CAD build for the part. Positions are in the model's coordinates, mm. Face numbers are marked on the shaded views. A direction names the side the tool comes from. Round coordinates to 2 decimals unless told otherwise and drop trailing zeros. Loops run counter-clockwise (first coordinate to the right, second up) from the corner with the lowest first, then second, coordinate; pieces in that order, holes last. Notation, with made-up numbers: M 87.5,22.25 L 135.5,22.25 A17 cw 135.5,29.25 Z; hole C 57.5,43.25 d3. An arc over 180 degrees is marked long. One line per item, written item: value. Start each with the question number.
from build123d import *

# Parameters (mm, degrees)
F1_DEPTH = 5
F2_DEPTH = 1


# Not quite as in the source:
# - a feature names something its author has since deleted; it is built from what else it names


with BuildPart() as f1:
    # F0 (on Front) → F1 (new body)
    with BuildSketch(Plane.XZ):
        with BuildLine():
            Line((1.2337693236, -4.7421317207), (20.7868759001, -2.4834859005))
            ThreePointArc((20.7868759001, -2.4834859005), (23, 0), (20.7868759001, 2.4834859005))
            Line((20.7868759001, 2.4834859005), (1.2337693236, 4.7421317207))
            ThreePointArc((1.2337693236, 4.7421317207), (-4.9, 0), (1.2337693236, -4.7421317207))
        make_face()
        with BuildLine():
            ThreePointArc((0, -3.5), (-3.5, 0), (0, 3.5))
            Line((0, 3.5), (16.1879612334, 1.8906799239))
            ThreePointArc((16.1879612334, 1.8906799239), (17.9, 0), (16.1879612334, -1.8906799239))
            Line((16.1879612334, -1.8906799239), (0, -3.5))
        make_face(mode=Mode.SUBTRACT)
    extrude(amount=F1_DEPTH)

    # F0 (on Front) → F2 (join)
    with BuildSketch(Plane.XZ):
        with BuildLine():
            Line((1.2337693236, -4.7421317207), (20.7868759001, -2.4834859005))
            ThreePointArc((20.7868759001, -2.4834859005), (23, 0), (20.7868759001, 2.4834859005))
            Line((20.7868759001, 2.4834859005), (1.2337693236, 4.7421317207))
            ThreePointArc((1.2337693236, 4.7421317207), (-4.9, 0), (1.2337693236, -4.7421317207))
        make_face()
        with BuildLine():
            ThreePointArc((0, -3.5), (-3.5, 0), (0, 3.5))
            Line((0, 3.5), (16.1879612334, 1.8906799239))
            ThreePointArc((16.1879612334, 1.8906799239), (17.9, 0), (16.1879612334, -1.8906799239))
            Line((16.1879612334, -1.8906799239), (0, -3.5))
        make_face(mode=Mode.SUBTRACT)
        with BuildLine():
            Line((16.1879612334, 1.8906799239), (0, 3.5))
            ThreePointArc((0, 3.5), (-3.5, 0), (0, -3.5))
            Line((0, -3.5), (16.1879612334, -1.8906799239))
            ThreePointArc((16.1879612334, -1.8906799239), (17.9, 0), (16.1879612334, 1.8906799239))
        make_face()
    extrude(amount=F2_DEPTH)


solid = f1.part
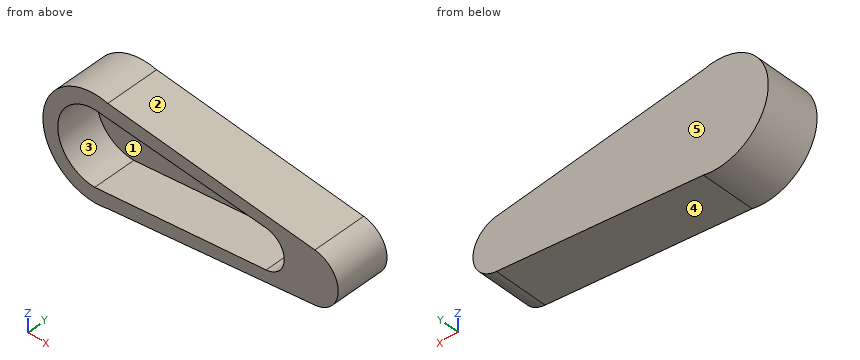
(1) Probe L1, parallel to Z at x = 2.75, y = -4.05; L2, parallel to Y at x = 1.5, z = -2; L3, parallel to Z at x = 6.5, y = -1.75. List the from-to ranges inside material, lowest first.
(2) Slice it at C-C, the plane x = 17.25. List the corners of the cut face in (y, z).
(3) Mould opens along X. For the marked faces 3, 4 and 5 say: pulls with the +X half, pulls with the -X half, needs draft (parallel to the pull), parting line crosses it, or undercut.
(4) Which spindle directions (+Z, -Z, +X, -X, +Y, -Y) get a long thin tool onto all of the face, cutting with end or side? Do the marked faces 1 and 2. Say none if no direction does.
(5) Slice it at D-D, the plane y = -0.55. List the corners of the cut face in (x, z).
(6) Slice it at B-B, the plane z = 0. List the corners of the cut face in (x, y).
(7) Flat gauge pins, fed straight in: P1, Ø2, axis at y = -4.5, z = 3, coming from the -X side; P2, Ø2, axis at x = 4, z = 0.5, coming from the -Y side. Where does each tip first touch, or does it go through?
(8) Slice it at A-A, the plane y = -2.35. List the corners of the cut face in (x, z).
Check result:
1. L1: z = -4.57 to -3.23, 3.23 to 4.57
1. L2: y = -1 to 0
1. L3: z = -4.13 to -2.85, 2.85 to 4.13
2. outline: M -5,-2.89 L 0,-2.89 L 0,2.89 L -5,2.89 L -5,1.43 L -1,1.43 L -1,-1.43 L -5,-1.43 Z
3. face 3: undercut
3. face 4: pulls with the +X half
3. face 5: needs draft
4. face 1: -Y
4. face 2: +Z, +X, +Y, -Y
5. outline: M 1.23,-4.74 L 20.79,-2.48 A2.5 ccw 20.79,2.48 L 1.23,4.74 A4.9 ccw long Z
6. outline: M -4.9,-5 L -3.5,-5 L -3.5,-1 L 17.9,-1 L 17.9,-5 L 23,-5 L 23,0 L -4.9,0 Z
7. P1: stops at x = -4.47
7. P2: stops at y = -1
8. outline: M 1.23,-4.74 L 20.79,-2.48 A2.5 ccw 20.79,2.48 L 1.23,4.74 A4.9 ccw long Z; hole M 0,-3.5 L 16.19,-1.89 A1.9 ccw 16.19,1.89 L 0,3.5 A3.5 ccw Z
